Source: CAD feature listing. Evaluate the final solid. Frame: model axes, mm. Round coordinates to 2 decimals unless told otherwise and drop trailing zeros. Order: outer loops, then holes, each group sorted by start corner. A loop starts at its lowest first (then second) coordinate and runs counter-clockwise, first axis right, second up. Notation, with made-up numbers: (-12.5, -16.75) -> (14.5, -16.75) arc R26 cw to (14.5, 21.25) -> close; hole circle Ø2 at (-6, 51). An arc over 180 degrees is marked (long way). Write item = value, one per line. Start each with the question number.
(1) Contact query for a flat-ended pin moving along its axis: pin 1 Ø8.5 at (x, z) = (9.7, 7.85) entering from +Y. Output: stop coordinate, or through.
(2) Cut plane B-B on z = 7.85. Return the cut outline in (x, y).
(3) Cut plane A-A on x = 9.7. Return the cut outline in (y, z).
(4) Ray query, line 1 (Z direction, x = 9.7, y = 1.15); line 2 (X direction, y = 1.05, z = 47.5); line 3 (X direction, y = 1.1, z = 7.85). Return the intervals inside material, ascending.
(5) Cut plane C-C on x = 98.05. Return the cut outline in (y, z), then the cut area to 3 significant figures.
from build123d import *

# Parameters (mm, degrees)
STOCK_BOTTOM_START        = 1
STOCK_BOTTOM_CASE_1_DEPTH = 0.2
CUT_EXTRUDE1_DEPTH        = 120.620159254
CUT_EXTRUDE1_DEPTH_BACK   = 120.620159254
SKETCH1_R                 = 3.75


# Read off the part's stored shape, not the designer's step: Stock-Bottom case-1
with BuildPart() as part:
    # Stock-Bottom case-1 outline → Stock-Bottom case-1 (new body)
    with BuildSketch(Plane(origin=(0, 0, 0), x_dir=(1, 0, 0), z_dir=(0, 1, 0)).offset(STOCK_BOTTOM_START)):
        with BuildLine():
            Line((94.55, 55.05), (-75.95, 55.05))
            Line((-75.95, 55.05), (-75.95, 47.6))
            ThreePointArc((-75.95, 47.6), (-79.45, 44.1), (-82.95, 47.6))
            Line((-82.95, 47.6), (-82.95, 55.05))
            Line((-82.95, 55.05), (-106.2, 55.05))
            Line((-106.2, 55.05), (-106.2, -55.05))
            Line((-106.2, -55.05), (-82.95, -55.05))
            Line((-82.95, -55.05), (-82.95, -47.6))
            ThreePointArc((-82.95, -47.6), (-79.45, -44.1), (-75.95, -47.6))
            Line((-75.95, -47.6), (-75.95, -55.05))
            Line((-75.95, -55.05), (94.55, -55.05))
            Line((94.55, -55.05), (94.55, -47.6))
            ThreePointArc((94.55, -47.6), (98.05, -44.1), (101.55, -47.6))
            Line((101.55, -47.6), (101.55, -55.05))
            Line((101.55, -55.05), (106.2, -55.05))
            Line((106.2, -55.05), (106.2, 55.05))
            Line((106.2, 55.05), (101.55, 55.05))
            Line((101.55, 55.05), (101.55, 47.6))
            ThreePointArc((101.55, 47.6), (98.05, 44.1), (94.55, 47.6))
            Line((94.55, 47.6), (94.55, 55.05))
        make_face()
    extrude(amount=STOCK_BOTTOM_CASE_1_DEPTH)

    # Sketch1 → Cut-Extrude1 (cut, two sides: drawn at the far end of the back side and taken through both)
    with BuildSketch(Plane(origin=(0, 1.2, 0), x_dir=(1, 0, 0), z_dir=(0, 1, 0)).offset(-CUT_EXTRUDE1_DEPTH_BACK)):
        with Locations(Location((9.7, -7.85, 0), (0, 0, 270))):
            Circle(SKETCH1_R)
    extrude(amount=CUT_EXTRUDE1_DEPTH + CUT_EXTRUDE1_DEPTH_BACK, mode=Mode.SUBTRACT)


solid = part.part
Evaluation:
q1.pin_1 = 1.2
q2.outline = (-106.2, 1) -> (5.95, 1) -> (5.95, 1.2) -> (-106.2, 1.2) -> close; (13.45, 1) -> (106.2, 1) -> (106.2, 1.2) -> (13.45, 1.2) -> close
q3.outline = (1, -55.05) -> (1.2, -55.05) -> (1.2, 4.1) -> (1, 4.1) -> close; (1, 11.6) -> (1.2, 11.6) -> (1.2, 55.05) -> (1, 55.05) -> close
q4.line_1 = -55.05 to 4.1, 11.6 to 55.05
q4.line_2 = -106.2 to -82.95, -75.95 to 94.55, 101.55 to 106.2
q4.line_3 = -106.2 to 5.95, 13.45 to 106.2
q5.outline = (1, -44.1) -> (1.2, -44.1) -> (1.2, 44.1) -> (1, 44.1) -> close
q5.area = 17.6 mm^2
